from build123d import *

# Parameters (mm, degrees)
EXTRUDE_1_DEPTH     = 5
CUT_EXTRUDE_1_DEPTH = 619.131054065
FILLET_1_R          = 5


with BuildPart() as part:
    # ｽｹｯﾁ2 → ﾎﾞｽ - 押し出し1 (new body)
    with BuildSketch(Plane.XY):
        Polygon((355, 0), (-355, 0), (-355, 20), (-262.5, 506), (262.5, 506), (355, 20), align=None)
    extrude(amount=EXTRUDE_1_DEPTH)

    # ｽｹｯﾁ3 → ｶｯﾄ - 押し出し1 (cut, through all)
    with BuildSketch(Plane.XY.offset(5)):
        Polygon((-262.5, 506), (-266.306584362, 486), (-220, 486), (-220, 506), align=None)
        Polygon((262.5, 506), (220, 506), (220, 486), (266.306584362, 486), align=None)
        with BuildLine():
            Line((5, 506), (-5, 506))
            Line((-5, 506), (-5, 496))
            ThreePointArc((-5, 496), (0, 491), (5, 496))
            Line((5, 496), (5, 506))
        make_face()
        with BuildLine():
            Line((-30, 10), (-30, 0))
            Line((-30, 0), (30, 0))
            Line((30, 0), (30, 10))
            ThreePointArc((30, 10), (28.535533906, 13.535533906), (25, 15))
            Line((25, 15), (-25, 15))
            ThreePointArc((-25, 15), (-28.535533906, 13.535533906), (-30, 10))
        make_face()
    extrude(amount=-CUT_EXTRUDE_1_DEPTH, mode=Mode.SUBTRACT)

    # ﾌｨﾚｯﾄ1
    fillet_1_edges = [part.edges().sort_by_distance(p)[0] for p in [
        (-355, 20, 2.5),
        (355, 20, 2.5),
        (355, 0, 2.5),
        (-355, 0, 2.5),
        (-220, 486, 2.5),
        (-266.306584362, 486, 2.5),
        (-220, 506, 2.5),
        (266.306584362, 486, 2.5),
        (220, 486, 2.5),
        (220, 506, 2.5),
        (-5, 506, 2.5),
        (5, 506, 2.5),
        (30, 0, 2.5),
        (-30, 0, 2.5),
    ]]
    fillet(fillet_1_edges, radius=FILLET_1_R)


solid = part.part
Geometry: final body of the model. Coordinates: model frame, mm. Round coordinates to 2 decimals unless told otherwise and drop trailing zeros. Loops run counter-clockwise (first coordinate to the right, second up) from the corner with the lowest first, then second, coordinate; pieces in that order, holes last. Notation, with made-up numbers: (13.5, 29) -> (19.5, 29) arc R21 ccw to (19.5, 38) -> close; hole circle Ø11 at (-8, 69.5). An arc over 180 degrees is marked (long way). One line per question, with ' | ' between items. Start each with the question number.
1. Contact query for flat-ended pins moving along their axis: pin 1 (2.5 mm diameter, centred on x = 243, z = 2.5, fed in from +Y); pin 2 (3 mm diameter, centred on y = 172.5, z = 1.5, fed in from +X). Output: stop coordinate, or through.
2. Section B-B on y = 335.5. Output: boundary loops of the cut face in (x, z).
3. Line query: line 1 along X through (y, z) = (47, 0.65); line 2 along Y through (x, z) = (-260, 4.5); line 3 along Y through (x, z) = (-12.5, 0.2). Output: solid intervals per line, ascending. Write a range as [from, to].
4. Section C-C on x = 305. Output: boundary loops of the cut face in (y, z), and give its area (3 significant figures).
Returned:
1) pin 1: stops at y = 486 | pin 2: stops at x = 326.26
2) outline: (-294.95, 0) -> (294.95, 0) -> (294.95, 5) -> (-294.95, 5) -> close
3) line 1: x = [-349.86, 349.86] | line 2: y = [0, 486] | line 3: y = [15, 506]
4) outline: (0, 0) -> (282.7, 0) -> (282.7, 5) -> (0, 5) -> close | area: 1,410 mm2
